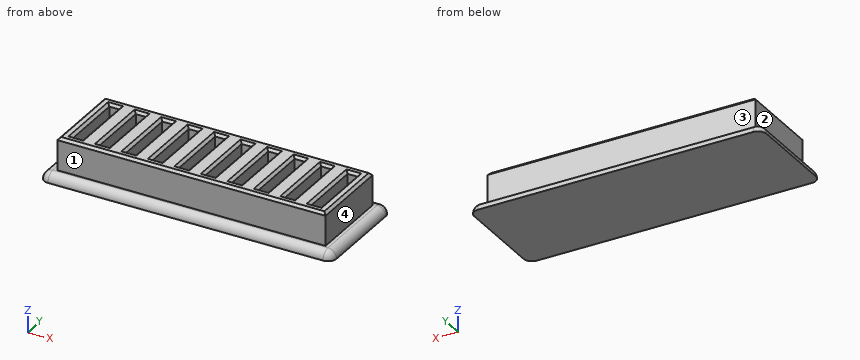
```python
from build123d import *

# Parameters (mm, degrees)
F0_W     = 156
F0_H     = 48
F1_DEPTH = 2
F2_W     = 156
F2_H     = 48
F2_W_2   = 5.7
F2_H_2   = 37.5
F3_DEPTH = 22
F0_W_2   = 170
F0_H_2   = 60
F4_DEPTH = 5
F5_R     = 4.99999
F6_SIZE  = 1.5


# Not quite as in the source:
# - a fillet or chamfer is up to 0.001 mm smaller than in the source, because OpenCascade refuses the exact size


with BuildPart() as f1:
    # F0 (on Top) → F1 (new body)
    with BuildSketch(Plane.XY):
        Rectangle(F0_W, F0_H)
    extrude(amount=F1_DEPTH)

    # F2 (on face) → F3 (join)
    with BuildSketch(Plane.XY.offset(2)):
        Rectangle(F2_W, F2_H)
        with Locations((-69.35, 0)):
            Rectangle(F2_W_2, F2_H_2, mode=Mode.SUBTRACT)
        with Locations((-53.95, 0)):
            Rectangle(F2_W_2, F2_H_2, mode=Mode.SUBTRACT)
        with Locations((-38.55, 0)):
            Rectangle(F2_W_2, F2_H_2, mode=Mode.SUBTRACT)
        with Locations((-23.15, 0)):
            Rectangle(F2_W_2, F2_H_2, mode=Mode.SUBTRACT)
        with Locations((-7.75, 0)):
            Rectangle(F2_W_2, F2_H_2, mode=Mode.SUBTRACT)
        with Locations((7.65, 0)):
            Rectangle(F2_W_2, F2_H_2, mode=Mode.SUBTRACT)
        with Locations((23.05, 0)):
            Rectangle(F2_W_2, F2_H_2, mode=Mode.SUBTRACT)
        with Locations((38.45, 0)):
            Rectangle(F2_W_2, F2_H_2, mode=Mode.SUBTRACT)
        with Locations((53.85, 0)):
            Rectangle(F2_W_2, F2_H_2, mode=Mode.SUBTRACT)
        with Locations((69.25, 0)):
            Rectangle(F2_W_2, F2_H_2, mode=Mode.SUBTRACT)
    extrude(amount=F3_DEPTH)

    # F0 (on Top) → F4 (join)
    with BuildSketch(Plane.XY):
        Rectangle(F0_W_2, F0_H_2)
        Rectangle(F0_W, F0_H, mode=Mode.SUBTRACT)
    extrude(amount=F4_DEPTH)

    # F5 (radius 5 in the source; OpenCascade refuses exactly that, so slightly less here)
    f5_edges = [f1.edges().sort_by_distance(p)[0] for p in [
        (0, -30, 5),
        (-85, 0, 5),
        (0, 30, 5),
        (85, 0, 5),
        (85, -30, 2.5),
        (85, 30, 2.5),
        (-85, -30, 2.5),
        (-85, 30, 2.5),
    ]]
    fillet(f5_edges, radius=F5_R)

    # F6
    f6_edges = [f1.edges().sort_by_distance(p)[0] for p in [
        (0, -24, 24),
        (-78, 0, 24),
        (0, 24, 24),
        (78, 0, 24),
        (-72.2, 0, 24),
        (-66.5, 0, 24),
        (-69.35, -18.75, 24),
        (-69.35, 18.75, 24),
        (-53.95, -18.75, 24),
        (-51.1, 0, 24),
        (-56.8, 0, 24),
        (-53.95, 18.75, 24),
        (-38.55, 18.75, 24),
        (-41.4, 0, 24),
        (-38.55, -18.75, 24),
        (-35.7, 0, 24),
        (-26, 0, 24),
        (-20.3, 0, 24),
        (-23.15, -18.75, 24),
        (-23.15, 18.75, 24),
        (-10.6, 0, 24),
        (-7.75, 18.75, 24),
        (-4.9, 0, 24),
        (-7.75, -18.75, 24),
        (7.65, -18.75, 24),
        (4.8, 0, 24),
        (10.5, 0, 24),
        (7.65, 18.75, 24),
        (20.2, 0, 24),
        (23.05, 18.75, 24),
        (25.9, 0, 24),
        (23.05, -18.75, 24),
        (38.45, -18.75, 24),
        (35.6, 0, 24),
        (41.3, 0, 24),
        (38.45, 18.75, 24),
        (51, 0, 24),
        (53.85, -18.75, 24),
        (56.7, 0, 24),
        (53.85, 18.75, 24),
        (66.4, 0, 24),
        (69.25, -18.75, 24),
        (72.1, 0, 24),
        (69.25, 18.75, 24),
    ]]
    chamfer(f6_edges, length=F6_SIZE)


solid = f1.part
```
Here's how the part is built. I have some questions about the finished solid (model axes, mm). Face numbers are marked on the shaded views. A direction names the side the tool comes from. Round coordinates to 2 decimals unless told otherwise and drop trailing zeros. Answer in a Markdown table with one row per item.
Item 1: If I drill on L1, parallel to Y at x = 36.5, z = 7.75; L2, parallel to Y at x = -76.5, z = 20.25; L3, parallel to Z at x = 7.5, y = -2, over which ranges is the centre line in solid material (lowest first)? Write a range as from..to.
A:
| item | result |
|---|---|
| L1 | y = -24..-18.75, 18.75..24 |
| L2 | y = -24..24 |
| L3 | z = 0..2 |
Item 2: I'm going to push flat-ended pins straight in: pin 1 (6.5 mm diameter, centred on x = -7.5, z = 12.5, fed in from -Y); pin 2 (3 mm diameter, centred on y = -19.5, z = 12.5, fed in from -X); pin 3 (6 mm diameter, centred on y = 1, z = 16, fed in from +X); pin 4 (2 mm diameter, centred on x = 56, y = 3.5, fed in from -Z). Where does each tip first touch, or does it pass through?
A:
| item | result |
|---|---|
| pin 1 | stops at y = -24 |
| pin 2 | stops at x = -78 |
| pin 3 | stops at x = 78 |
| pin 4 | stops at z = 0 |
Item 3: For the marked faces 1, 2, 3 and 4, which set-ups out of +Z, -Z, +X, -X, +Y, -Y let a thin tool reach every point of the face, with its end or its side?
A:
| item | result |
|---|---|
| face 1 | +Z, +X, -X, -Y |
| face 2 | +Z, -X, +Y, -Y |
| face 3 | +Z, +X, -X, +Y |
| face 4 | +Z, +X, +Y, -Y |
Item 4: Imagine slicing it at B-B, the plane z = 15.5. State how many separate pieces and enclosed holes the cut face has, and give its area (3 significant figures).
A:
| item | result |
|---|---|
| separate pieces | 1 |
| enclosed holes | 10 |
| area | 5,350 mm2 |
